The listing builds one solid part. Answer for the finished solid, in the listing's coordinates (mm). Face numbers are marked on the shaded views. A direction names the side the tool comes from. Coordinates: 2 decimals unless noted, no trailing zeros. Write each loop counter-clockwise with the first axis right and the second up, starting at its lowest first coordinate (ties: lowest second). Pieces come first, ordered by that corner, then holes.
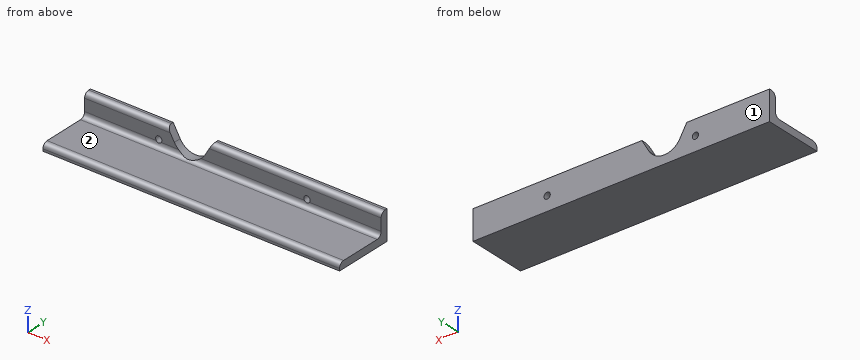
from build123d import *

# Parameters (mm, degrees)
F1_DEPTH = 127
F2_R     = 1.3462
F3_DEPTH = 25.2994
F5_DEPTH = 25.2994


with BuildPart() as f1:
    # F0 (on Right) → F1 (new body)
    with BuildSketch(Plane.YZ):
        with BuildLine():
            Line((-10.285505, -7.297242), (-10.285505, -8.262442))
            Line((-10.285505, -8.262442), (15.012895, -8.262442))
            Line((15.012895, -8.262442), (15.012895, 4.335958))
            Line((15.012895, 4.335958), (14.047695, 4.335958))
            ThreePointArc((14.047695, 4.335958), (12.521052, 3.703602), (11.888695, 2.176958))
            Line((11.888695, 2.176958), (11.888695, -2.979242))
            ThreePointArc((11.888695, -2.979242), (11.256339, -4.505885), (9.729695, -5.138242))
            Line((9.729695, -5.138242), (-8.126505, -5.138242))
            ThreePointArc((-8.126505, -5.138242), (-9.653148, -5.770598), (-10.285505, -7.297242))
        make_face()
    extrude(amount=F1_DEPTH)

    # F2 (on face) → F3 (cut, through all)
    with BuildSketch(Plane(origin=(0, 15.012895, 0), x_dir=(-1, 0, 0), z_dir=(0, 1, 0))):
        with Locations((-31.75, -2.166442)):
            Circle(F2_R)
        with Locations((-95.25, -2.166442)):
            Circle(F2_R)
    extrude(amount=-F3_DEPTH, mode=Mode.SUBTRACT)

    # F4 (on face) → F5 (cut, through all)
    with BuildSketch(Plane(origin=(0, 15.012895, 0), x_dir=(-1, 0, 0), z_dir=(0, 1, 0))):
        with BuildLine():
            Line((-54.656256, 4.335958), (-51.635329, -0.896442))
            ThreePointArc((-51.635329, -0.896442), (-45.036215, -4.706442), (-38.437102, -0.896442))
            Line((-38.437102, -0.896442), (-35.416174, 4.335958))
            Line((-35.416174, 4.335958), (-54.656256, 4.335958))
        make_face()
    extrude(amount=-F5_DEPTH, mode=Mode.SUBTRACT)


solid = f1.part
1. Section D-D on y = -3 is taken. Give the vertices of the cut face in (x, z).
Results found:
outline: (0, -8.26) - (127, -8.26) - (127, -5.14) - (0, -5.14) - close
2. Flat-ended cylindrical pins translate along their axes: P1, Ø1.5, axis at x = 53.5, y = 5.5, coming from the +Z side; P2, Ø1.5, axis at x = 23, z = 0.5, coming from the -Y side; P3, Ø4.5, axis at x = 31.75, z = -2.17, coming from the -Y side. Find the tip coordinate at first contact, or state that the pin passes through.
Results found:
P1: stops at z = -5.14
P2: stops at y = 11.89
P3: stops at y = 11.34
3. Section A-A on x = 95.25 is taken. Give the vertices of the cut face in (y, z), then the cut area to 3 significant figures.
Results found:
outline: (-10.29, -8.26) - (15.01, -8.26) - (15.01, -3.51) - (11.82, -3.51) arc R2.16 cw to (9.73, -5.14) - (-8.13, -5.14) arc R2.16 ccw to (-10.29, -7.3) - close; (11.89, -0.82) - (15.01, -0.82) - (15.01, 4.34) - (14.05, 4.34) arc R2.16 ccw to (11.89, 2.18) - close
area: 99.2 mm2
4. Find the intervals of material crossed by L1, parallel to Z at x = 31.75, y = 14.2; L2, parallel to Z at x = 74, y = 6.5; L3, parallel to Y at x = 30.5, z = -0.5, in increasing order.
Results found:
L1: z = -8.26 to -3.51, -0.82 to 4.34
L2: z = -8.26 to -5.14
L3: y = 11.89 to 15.01
5. Section C-C on x = 109 is taken. Give the vertices of the cut face in (y, z).
Results found:
outline: (-10.29, -8.26) - (15.01, -8.26) - (15.01, 4.34) - (14.05, 4.34) arc R2.16 ccw to (11.89, 2.18) - (11.89, -2.98) arc R2.16 cw to (9.73, -5.14) - (-8.13, -5.14) arc R2.16 ccw to (-10.29, -7.3) - close
6. Section B-B on z = 3.25 is taken. Give the vertices of the cut face in (x, y), then the cut area to 3 significant figures.
Results found:
outline: (0, 12.17) - (36.04, 12.17) - (36.04, 15.01) - (0, 15.01) - close; (54.03, 12.17) - (127, 12.17) - (127, 15.01) - (54.03, 15.01) - close
area: 309 mm2
7. A tool of negligible diameter and unlimited length cuts with its end or side. For the marked faces 1 and 2, from which of +Z, -Z, +X, -X, +Y, -Y can it reach the whole face along a straight path? Write none if from no direction.
Results found:
face 1: +Z, -Z, +X, -X, +Y
face 2: +Z, +X, -X, -Y
